Verification items for the finished model (mm, model axes). Face numbers are marked on the shaded views. A direction names the side the tool comes from. Give positions to 0.01 mm unless a question says otherwise; leave off trailing zeros. Write each loop counter-clockwise with the first axis right and the second up, starting at its lowest first coordinate (ties: lowest second). Pieces come first, ordered by that corner, then holes.
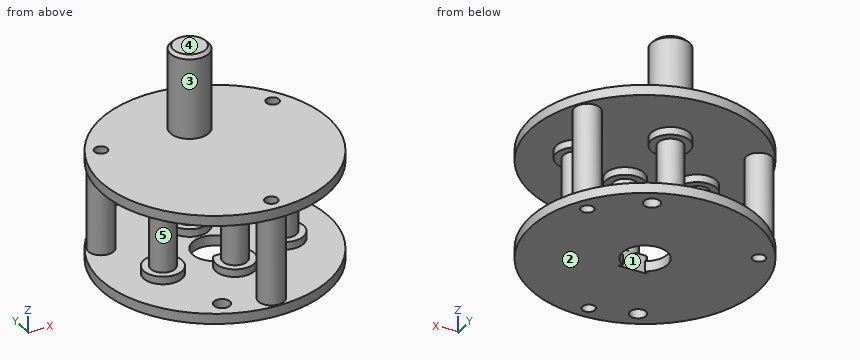
from build123d import *

# Parameters (mm, degrees)
SKETCH_1_R          = 17.75
EXTRUDE_1_DEPTH     = 1.6
SKETCH_2_R          = 2
EXTRUDE_2_DEPTH     = 13.8
EXTRUDE_START       = 1.6
SKETCH_3_R          = 17.75
EXTRUDE_3_DEPTH     = 1.6
CUT_EXTRUDE_2_REACH = 32.317
SKETCH_5_R          = 3.5
SKETCH_5_R_2        = 1
SKETCH_6_R          = 6
EXTRUDE_4_DEPTH     = 10
SKETCH_7_R          = 3
EXTRUDE_5_DEPTH     = 15
CHAMFER_1_SIZE      = 0.5
CUT_EXTRUDE_START   = -12
CUT_EXTRUDE_3_DEPTH = 12
SKETCH_10_R         = 3
EXTRUDE_6_DEPTH     = 2.8
EXTRUDE_7_REACH     = 39.456
SKETCH_13_R         = 1.9
CUT_EXTRUDE_4_REACH = 50.93
CUT_EXTRUDE_5_REACH = 50.93
SKETCH_17_R         = 1.25
CHAMFER_2_SIZE      = 0.5
EXTRUDE_START_2     = 1.2
SKETCH_19_R         = 3
EXTRUDE_8_DEPTH     = 1.2
EXTRUDE_9_REACH     = 39.456
SKETCH_20_R         = 1.9
SKETCH_21_R         = 3
EXTRUDE_10_DEPTH    = 1.2
CUT_EXTRUDE_START_2 = -10
SKETCH_23_R         = 6
SKETCH_23_R_2       = 3
CUT_EXTRUDE_7_DEPTH = 10
SKETCH_24_R         = 3
CUT_EXTRUDE_8_DEPTH = 12
CHAMFER_3_SIZE      = 0.5


with BuildPart() as part:
    # Sketch 1 → Extrude 1 (new body)
    with BuildSketch(Plane.XY):
        Circle(SKETCH_1_R)
    extrude(amount=EXTRUDE_1_DEPTH)

    # Sketch 2 → Extrude 2 (add)
    with BuildSketch(Plane(origin=(0, 0, 0), x_dir=(-1, 0, 0), z_dir=(0, 0, -1))):
        with Locations(Location((0, -15.5, 0), (0, 0, 180))):
            Circle(SKETCH_2_R)
        with Locations(Location((-13.423393759, 7.75, 0), (0, 0, 180))):
            Circle(SKETCH_2_R)
        with Locations(Location((13.423393759, 7.75, 0), (0, 0, 180))):
            Circle(SKETCH_2_R)
    extrude(amount=EXTRUDE_2_DEPTH)

    # Sketch 3 → Extrude 3 (add)
    with BuildSketch(Plane(origin=(0, 0, -13.8), x_dir=(-1, 0, 0), z_dir=(0, 0, -1)).offset(EXTRUDE_START)):
        with Locations(Location((0, 0, 0), (0, 0, 180))):
            Circle(SKETCH_3_R)
    extrude(amount=-EXTRUDE_3_DEPTH)

    # Sketch 5 → Cut-Extrude 2 (cut, up to next)
    with BuildSketch(Plane(origin=(0, 0, -15.4), x_dir=(-1, 0, 0), z_dir=(0, 0, -1)), mode=Mode.PRIVATE) as cut_extrude_2_sk1:
        Circle(SKETCH_5_R)
    cut_extrude_2_tool1 = extrude(cut_extrude_2_sk1.sketch, amount=-CUT_EXTRUDE_2_REACH, mode=Mode.PRIVATE) & part.part
    # Sketch 5 → Cut-Extrude 2 (cut, up to next)
    with BuildSketch(Plane(origin=(0, 0, -15.4), x_dir=(-1, 0, 0), z_dir=(0, 0, -1)), mode=Mode.PRIVATE) as cut_extrude_2_sk2:
        with Locations((-13.423393759, 7.75)):
            Circle(SKETCH_5_R_2)
    cut_extrude_2_tool2 = extrude(cut_extrude_2_sk2.sketch, amount=-CUT_EXTRUDE_2_REACH, mode=Mode.PRIVATE) & part.part
    # Sketch 5 → Cut-Extrude 2 (cut, up to next)
    with BuildSketch(Plane(origin=(0, 0, -15.4), x_dir=(-1, 0, 0), z_dir=(0, 0, -1)), mode=Mode.PRIVATE) as cut_extrude_2_sk3:
        with Locations((13.423393759, 7.75)):
            Circle(SKETCH_5_R_2)
    cut_extrude_2_tool3 = extrude(cut_extrude_2_sk3.sketch, amount=-CUT_EXTRUDE_2_REACH, mode=Mode.PRIVATE) & part.part
    # Sketch 5 → Cut-Extrude 2 (cut, up to next)
    with BuildSketch(Plane(origin=(0, 0, -15.4), x_dir=(-1, 0, 0), z_dir=(0, 0, -1)), mode=Mode.PRIVATE) as cut_extrude_2_sk4:
        with Locations((0, -15.5)):
            Circle(SKETCH_5_R_2)
    cut_extrude_2_tool4 = extrude(cut_extrude_2_sk4.sketch, amount=-CUT_EXTRUDE_2_REACH, mode=Mode.PRIVATE) & part.part
    add(cut_extrude_2_tool1.solids().sort_by_distance((0, 0, -15.4))[0], mode=Mode.SUBTRACT)
    add(cut_extrude_2_tool2.solids().sort_by_distance((13.423394, 7.75, -15.4))[0], mode=Mode.SUBTRACT)
    add(cut_extrude_2_tool3.solids().sort_by_distance((-13.423394, 7.75, -15.4))[0], mode=Mode.SUBTRACT)
    add(cut_extrude_2_tool4.solids().sort_by_distance((0, -15.5, -15.4))[0], mode=Mode.SUBTRACT)

    # Sketch 6 → Extrude 4 (add)
    with BuildSketch(Plane.XY.offset(1.6)):
        with Locations((0, 7)):
            Circle(SKETCH_6_R)
    extrude(amount=EXTRUDE_4_DEPTH)

    # Sketch 7 → Extrude 5 (add)
    with BuildSketch(Plane.XY.offset(11.6)):
        with Locations((0, 7)):
            Circle(SKETCH_7_R)
    extrude(amount=EXTRUDE_5_DEPTH)

    # Chamfer 1
    chamfer_1_edges = [part.edges().sort_by_distance(p)[0] for p in [
        (-3, 7, 26.6),
    ]]
    chamfer(chamfer_1_edges, length=CHAMFER_1_SIZE)

    # Sketch 8 → Cut-Extrude 3 (cut)
    with BuildSketch(Plane.XY.offset(26.6).offset(CUT_EXTRUDE_START)):
        with BuildLine():
            Line((1.658312395, 9.5), (-1.658312395, 9.5))
            ThreePointArc((-1.658312395, 9.5), (0, 10), (1.658312395, 9.5))
        make_face()
    extrude(amount=CUT_EXTRUDE_3_DEPTH, mode=Mode.SUBTRACT)

    # Sketch 10 → Extrude 6 (add)
    with BuildSketch(Plane.XY.offset(1.6)):
        with Locations((0, -5.5)):
            Circle(SKETCH_10_R)
        with Locations((9.5, -2.377501001)):
            Circle(SKETCH_10_R)
        with Locations((-9.5, -2.377501001)):
            Circle(SKETCH_10_R)
    extrude_6 = extrude(amount=-EXTRUDE_6_DEPTH)

    # Mirror 1: Extrude 6 across plane
    add(extrude_6.mirror(Plane.XY.offset(-6.9)))

    # Sketch 13 → Extrude 7 (add, up to next)
    with BuildSketch(Plane(origin=(0, 0, -1.2), x_dir=(-1, 0, 0), z_dir=(0, 0, -1)), mode=Mode.PRIVATE) as extrude_7_sk1:
        with Locations(Location((-9.5, -2.377501001, 0), (0, 0, 180))):
            Circle(SKETCH_13_R)
    extrude_7_tool1 = extrude(extrude_7_sk1.sketch, amount=EXTRUDE_7_REACH, mode=Mode.PRIVATE) - part.part
    # Sketch 13 → Extrude 7 (add, up to next)
    with BuildSketch(Plane(origin=(0, 0, -1.2), x_dir=(-1, 0, 0), z_dir=(0, 0, -1)), mode=Mode.PRIVATE) as extrude_7_sk2:
        with Locations(Location((0, -5.5, 0), (0, 0, 180))):
            Circle(SKETCH_13_R)
    extrude_7_tool2 = extrude(extrude_7_sk2.sketch, amount=EXTRUDE_7_REACH, mode=Mode.PRIVATE) - part.part
    # Sketch 13 → Extrude 7 (add, up to next)
    with BuildSketch(Plane(origin=(0, 0, -1.2), x_dir=(-1, 0, 0), z_dir=(0, 0, -1)), mode=Mode.PRIVATE) as extrude_7_sk3:
        with Locations(Location((9.5, -2.377501001, 0), (0, 0, 180))):
            Circle(SKETCH_13_R)
    extrude_7_tool3 = extrude(extrude_7_sk3.sketch, amount=EXTRUDE_7_REACH, mode=Mode.PRIVATE) - part.part
    add(extrude_7_tool1.solids().sort_by_distance((9.5, -2.377501, -1.2))[0])
    add(extrude_7_tool2.solids().sort_by_distance((0, -5.5, -1.2))[0])
    add(extrude_7_tool3.solids().sort_by_distance((-9.5, -2.377501, -1.2))[0])

    # Sketch 15 → Cut-Extrude 4 (cut, up to next)
    with BuildSketch(Plane(origin=(0, 0, -15.4), x_dir=(-1, 0, 0), z_dir=(0, 0, -1)), mode=Mode.PRIVATE) as cut_extrude_4_sk1:
        with BuildLine():
            Line((2.236067977, -3.5), (-2.236067977, -3.5))
            ThreePointArc((-2.236067977, -3.5), (-1.99347124, -3.258109634), (-1.724878724, -3.045454545))
            ThreePointArc((-1.724878724, -3.045454545), (0, -2.5), (1.724878724, -3.045454545))
            ThreePointArc((1.724878724, -3.045454545), (1.99347124, -3.258109634), (2.236067977, -3.5))
        make_face()
    cut_extrude_4_tool1 = extrude(cut_extrude_4_sk1.sketch, amount=-CUT_EXTRUDE_4_REACH, mode=Mode.PRIVATE) & part.part
    add(cut_extrude_4_tool1.solids().sort_by_distance((0, -3.093671, -15.4))[0], mode=Mode.SUBTRACT)

    # Sketch 17 → Cut-Extrude 5 (cut, up to next)
    with BuildSketch(Plane(origin=(0, 0, -15.4), x_dir=(-1, 0, 0), z_dir=(0, 0, -1)), mode=Mode.PRIVATE) as cut_extrude_5_sk1:
        with Locations((-6.569553896, 13.48484192)):
            Circle(SKETCH_17_R)
    cut_extrude_5_tool1 = extrude(cut_extrude_5_sk1.sketch, amount=-CUT_EXTRUDE_5_REACH, mode=Mode.PRIVATE) & part.part
    # Sketch 17 → Cut-Extrude 5 (cut, up to next)
    with BuildSketch(Plane(origin=(0, 0, -15.4), x_dir=(-1, 0, 0), z_dir=(0, 0, -1)), mode=Mode.PRIVATE) as cut_extrude_5_sk2:
        with Locations((6.569553896, -13.48484192)):
            Circle(SKETCH_17_R)
    cut_extrude_5_tool2 = extrude(cut_extrude_5_sk2.sketch, amount=-CUT_EXTRUDE_5_REACH, mode=Mode.PRIVATE) & part.part
    add(cut_extrude_5_tool1.solids().sort_by_distance((6.569554, 13.484842, -15.4))[0], mode=Mode.SUBTRACT)
    add(cut_extrude_5_tool2.solids().sort_by_distance((-6.569554, -13.484842, -15.4))[0], mode=Mode.SUBTRACT)

    # Chamfer 2
    chamfer_2_edges = [part.edges().sort_by_distance(p)[0] for p in [
        (-6, 7, 11.6),
    ]]
    chamfer(chamfer_2_edges, length=CHAMFER_2_SIZE)

    # Sketch 19 → Extrude 8 (add)
    with BuildSketch(Plane(origin=(0, 0, 0), x_dir=(-1, 0, 0), z_dir=(0, 0, -1)).offset(EXTRUDE_START_2)):
        with Locations(Location((0, 7, 0), (0, 0, 56.442690238))):
            Circle(SKETCH_19_R)
    extrude(amount=-EXTRUDE_8_DEPTH)

    # Sketch 20 → Extrude 9 (add, up to next)
    with BuildSketch(Plane(origin=(0, 0, -1.2), x_dir=(-1, 0, 0), z_dir=(0, 0, -1)), mode=Mode.PRIVATE) as extrude_9_sk1:
        with Locations(Location((0, 7, 0), (0, 0, 180))):
            Circle(SKETCH_20_R)
    extrude_9_tool1 = extrude(extrude_9_sk1.sketch, amount=EXTRUDE_9_REACH, mode=Mode.PRIVATE) - part.part
    add(extrude_9_tool1.solids().sort_by_distance((0, 7, -1.2))[0])

    # Sketch 21 → Extrude 10 (add)
    with BuildSketch(Plane.XY.offset(-13.8)):
        with Locations(Location((0, 7, 0), (0, 0, 123.557309762))):
            Circle(SKETCH_21_R)
    extrude(amount=EXTRUDE_10_DEPTH)

    # Sketch 23 → Cut-Extrude 7 (cut)
    with BuildSketch(Plane.XY.offset(11.6).offset(CUT_EXTRUDE_START_2)):
        with Locations((0, 7)):
            Circle(SKETCH_23_R)
        with Locations((0, 7)):
            Circle(SKETCH_23_R_2, mode=Mode.SUBTRACT)
    extrude(amount=CUT_EXTRUDE_7_DEPTH, mode=Mode.SUBTRACT)

    # Sketch 24 → Cut-Extrude 8 (cut)
    with BuildSketch(Plane.XY.offset(26.6).offset(CUT_EXTRUDE_START)):
        with Locations((0, 7)):
            Circle(SKETCH_24_R)
    extrude(amount=CUT_EXTRUDE_8_DEPTH, mode=Mode.SUBTRACT)

    # Chamfer 3
    chamfer_3_edges = [part.edges().sort_by_distance(p)[0] for p in [
        (-3, 7, 14.6),
    ]]
    chamfer(chamfer_3_edges, length=CHAMFER_3_SIZE)


solid = part.part
Item 1: Sectioned sample at A-A on y = -15.5. Record the cut outline in (x, z).
Answer key:
outline: (-8.65, -15.4) - (-1, -15.4) - (-1, 1.6) - (-8.65, 1.6) - (-8.65, 0) - (-2, 0) - (-2, -13.8) - (-8.65, -13.8) - close; (1, -15.4) - (8.65, -15.4) - (8.65, -13.8) - (2, -13.8) - (2, 0) - (8.65, 0) - (8.65, 1.6) - (1, 1.6) - close
Item 2: Scan lines: line 1 along Y through (x, z) = (0, -4); line 2 along Z through (x, y) = (-12, -3); line 3 along Z through (x, y) = (1.5, -13). Record each from-to range of solid material in increasing order.
Answer key:
line 1: y = -17.5 to -16.5, -14.5 to -13.5, -7.4 to -3.6, 5.1 to 8.9
line 2: z = -15.4 to -12.6, -1.2 to 1.6
line 3: z = -15.4 to -13.8, 0 to 1.6
Item 3: Sectioned sample at B-B on x = 0. State how many separate pieces and enclosed holes the cut face has, then the cut area to 3 significant figures.
Answer key:
separate pieces: 2
enclosed holes: 1
area: 316 mm2
Item 4: Depth check by flat-ended pin: pin 1 (3 mm diameter, centred on x = -2.5, z = -6.5, fed in from +Y); pin 2 (6 mm diameter, centred on y = -6, z = -9, fed in from +X); pin 3 (1.8 mm diameter, centred on x = 0, y = -15.5, fed in from -Z); pin 4 (12 mm diameter, centred on x = 8.5, y = -11.5, fed in from +Z). Enter the tip coordinate at first touch or a pass-through.
Answer key:
pin 1: stops at y = 8.62
pin 2: stops at x = 11.3
pin 3: passes through
pin 4: stops at z = 1.6
Item 5: Release check for a two-part mould opening along X. For the marked faces 1, 2 and 3 record: released by +X, released by -X, zero draft, split by the parting line, or undercut.
Answer key:
face 1: undercut
face 2: zero draft
face 3: split by the parting line
Item 6: Set-up check for the marked faces 4 and 5: record each of +Z, -Z, +X, -X, +Y, -Y from which the full face is reachable in a straight line by a thin tool's end or side.
Answer key:
face 4: +Z, +X, -X, +Y, -Y
face 5: none
